from build123d import *

# Parameters (mm, degrees)
SKETCH_R              = 25
PAD_DEPTH             = 1
SKETCH001_R           = 19
PAD001_DEPTH          = 8
POCKET_DEPTH          = 8
POLARPATTERN_COUNT    = 4
POCKET001_DEPTH       = 1
POLARPATTERN001_COUNT = 11


with BuildPart() as part:
    # Sketch → Pad (new body)
    with BuildSketch(Plane.XY):
        Circle(SKETCH_R)
    extrude(amount=PAD_DEPTH)

    # Sketch001 (on Face3 of Pad) → Pad001 (join)
    with BuildSketch(Plane.XY.offset(1)):
        Circle(SKETCH001_R)
    extrude(amount=PAD001_DEPTH)

    # Sketch002 (on Face5 of Pad001) → Pocket (cut)
    with BuildSketch(Plane.XY.offset(9)):
        with BuildLine():
            ThreePointArc((-1, 17.972201), (-12.727922, 12.727922), (-17.972201, 1))
            Line((-1, 1), (-17.972201, 1))
            Line((-1, 1), (-1, 17.972201))
        make_face()
    pocket = extrude(amount=-POCKET_DEPTH, mode=Mode.SUBTRACT)

    # PolarPattern: Pocket ×4 about axis
    polarpattern_axis = Axis((0, 0, 9), (0, 0, 1))
    for i in range(1, POLARPATTERN_COUNT):
        add(pocket.rotate(polarpattern_axis, i * 360 / POLARPATTERN_COUNT), mode=Mode.SUBTRACT)

    # Sketch003 (on Face2 of PolarPattern) → Pocket001 (cut)
    with BuildSketch(Plane(origin=(0, 0, 0), x_dir=(1, 0, 0), z_dir=(0, 0, -1))):
        with BuildLine():
            Line((0.558896, 6.977653), (1.396138, 19.95121))
            ThreePointArc((7.893916, 18.376237), (4.711307, 19.43717), (1.396138, 19.95121))
            Line((2.669717, 6.470905), (7.893916, 18.376237))
            ThreePointArc((2.669717, 6.470905), (1.63407, 6.806601), (0.558896, 6.977653))
        make_face()
    pocket001 = extrude(amount=-POCKET001_DEPTH, mode=Mode.SUBTRACT)

    # PolarPattern001: Pocket001 ×11 about axis
    polarpattern001_axis = Axis((0, 0, 0), (0, 0, -1))
    for i in range(1, POLARPATTERN001_COUNT):
        add(pocket001.rotate(polarpattern001_axis, i * 360 / POLARPATTERN001_COUNT), mode=Mode.SUBTRACT)


solid = part.part
Geometry: final body of the model. Coordinates: model frame, mm. A direction names the side the tool comes from. Round coordinates to 2 decimals unless told otherwise and drop trailing zeros. Loops run counter-clockwise (first coordinate to the right, second up) from the corner with the lowest first, then second, coordinate; pieces in that order, holes last.
Q1. Section A-A on z = 4.75. Return loops of the section in (x, y), plus the area to 3 significant figures.
Q2. Pin query (flat end, axial travel): P1, Ø1, axis at x = 16, y = -1, coming from the -Z side; P2, Ø4, axis at x = 9, z = 6.5, coming from the +Y side; P3, Ø2.5, axis at x = -11.5, z = 6, coming from the +Y side. Return the tip coordinate at first contact, or that it passes through.
Q3. Access query for faces 3 (the flat face through (4, -18, 1)), 4 (the flat face through (9, 1, 5)), 5 (the cylindrical face through (-5.5, -4.33, 0.49)). Directions: +Z, -Z, +X, -X, +Y, -Y. A direction counts if a zero-diameter tool reaches every point of the face in a straight line with its end or side. Return the directions, or none.
Q4. Pull-direction query (X, two-part tool) for faces 1 (the flat face through (-1.556, 13.318, 0.493)), 2 (the flat face through (0, 1, 9)); classes: released by +X, released by -X, zero draft, split by the parting line, or undercut.
Q5. Material intervals for L1, parallel to Y at x = -3.5, z = 5.5; L2, parallel to Y at x = -10.5, z = 3.5; L3, parallel to X at y = 15.5, z = 4, sorted ascending.
Evaluation:
1. outline: circle Ø38 at (0, 0); hole (-17.97, -1) arc R18 ccw to (-1, -17.97) - (-1, -1) - close; hole (-17.97, 1) - (-1, 1) - (-1, 17.97) arc R18 ccw to start; hole (1, -17.97) arc R18 ccw to (17.97, -1) - (1, -1) - close; hole (1, 1) - (17.97, 1) arc R18 ccw to (1, 17.97) - close
1. area: 256 mm2
2. P1: stops at z = 1
2. P2: stops at y = 17.66
2. P3: stops at y = 16
3. face 3: -Z
3. face 4: +Z
3. face 5: +Z, -Z
4. face 1: undercut
4. face 2: zero draft
5. L1: y = -18.67 to -17.66, -1 to 1, 17.66 to 18.67
5. L2: y = -15.84 to -14.62, -1 to 1, 14.62 to 15.84
5. L3: x = -10.99 to -9.15, -1 to 1, 9.15 to 10.99
